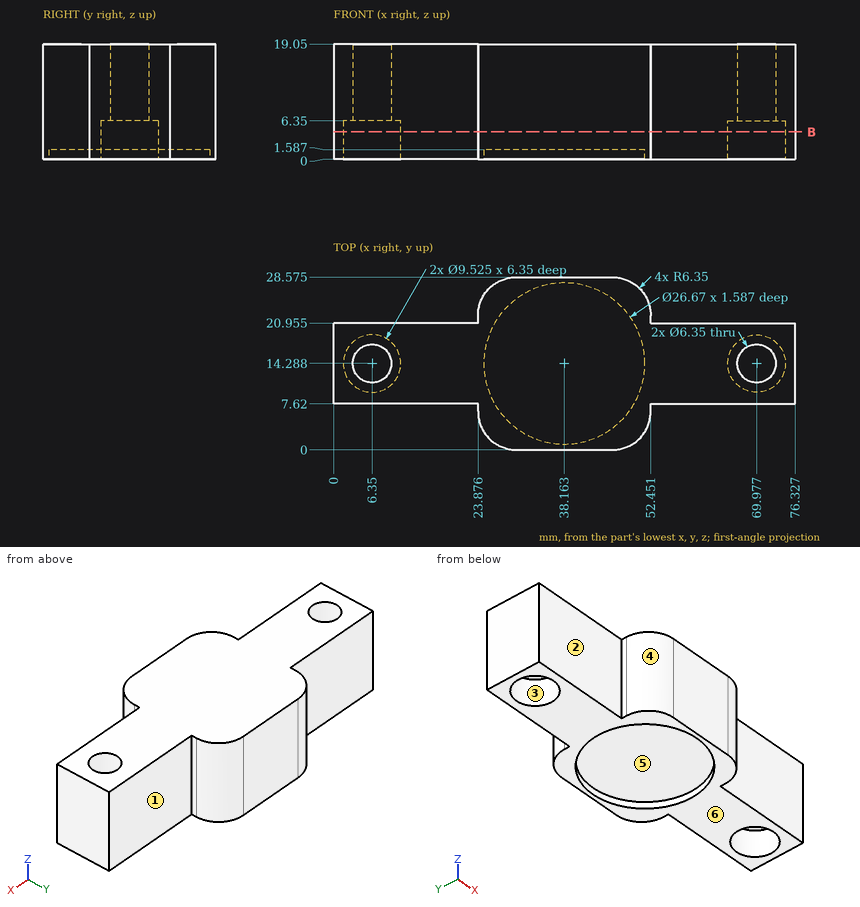
Input: dimensioned drawing with shaded views. Units: mm. Origin: part minimum x, y, z. A direction names the side the tool comes from. Coordinates: 2 decimals unless noted, no trailing zeros.
1. Access query for the marked faces 1, 2 and 3. Directions: +Z, -Z, +X, -X, +Y, -Y. A direction counts if a zero-diameter tool reaches every point of the face in a straight line with its end or side. Return the directions, or none.
Checked values:
face 1: +Z, -Z, +X, +Y
face 2: +Z, -Z, -X, -Y
face 3: -Z
2. Ray query, line 1 along Y through (x, z) = (6.35, 14.75) (1 decimal); line 2 along X through (y, z) = (17, 13.25) (1 decimal); line 3 along Y through (x, z) = (12, 6.25) (1 decimal). Return the intervals inside material, ascending.
Checked values:
line 1: y = 7.6 to 11.1, 17.5 to 21
line 2: x = 0 to 4.7, 8 to 68.3, 71.6 to 76.3
line 3: y = 7.6 to 21
3. Draft query along X for the marked faces 4, 5 and 6. Return one class per face: +X half, -X half, draft (parallel to the pull), parting line (faces both ways), or undercut.
Checked values:
face 4: -X half
face 5: undercut
face 6: draft
4. Cut plane B-B, the plane z = 4.5. Count the separate pieces of the cut face and the enclosed holes in it, plus the area to 3 significant figures.
Checked values:
separate pieces: 1
enclosed holes: 2
area: 1,280 mm2
5. Contact query for flat-ended pins moving along their axis: P1, Ø1, axis at x = 62, z = 10, coming from the -Y side; P2, Ø3, axis at x = 70, y = 14, coming from the -Z side; P3, Ø5.5, axis at x = 59, z = 5, coming from the +Y side (1 decimal); P4, Ø13.5, axis at x = 38.5, y = 10.5, coming from the -Z side. Output: stop coordinate, or through.
Checked values:
P1: stops at y = 7.62
P2: passes through
P3: stops at y = 21
P4: stops at z = 1.59
